```python
from build123d import *

# Parameters (mm, degrees)
F0_W     = 30
F0_H     = 30
F1_DEPTH = 15
F2_R     = 2
F4_R     = 1.75


with BuildPart() as f1:
    # F0 (on Top) → F1 (new body, symmetric)
    with BuildSketch(Plane.XY):
        Rectangle(F0_W, F0_H)
    extrude(amount=F1_DEPTH, both=True)

    # F2
    f2_edges = [f1.edges().sort_by_distance(p)[0] for p in [
        (15, 0, 15),
        (0, 15, 15),
        (-15, 0, 15),
        (0, -15, 15),
        (0, -15, -15),
        (15, -15, 0),
        (-15, -15, 0),
        (15, 0, -15),
        (15, 15, 0),
        (0, 15, -15),
        (-15, 15, 0),
        (-15, 0, -15),
    ]]
    fillet(f2_edges, radius=F2_R)

    # F5: sweep along a path in F3
    with BuildLine(Plane.XY) as f5_path:
        CenterArc((0, 19), 7, 0, 360)
    # F4 (on face) → F5 (sweep)
    with BuildSketch(Plane(origin=(0, 15, 0), x_dir=(-1, 0, 0), z_dir=(0, 1, 0))):
        with Locations((5.6, 0)):
            Circle(F4_R)
    sweep(path=f5_path.line)


solid = f1.part
```
Geometry: final body of the model. Coordinates: model frame, mm. Coordinates: 2 decimals unless noted, no trailing zeros. Write each loop counter-clockwise with the first axis right and the second up, starting at its lowest first coordinate (ties: lowest second). Pieces come first, ordered by that corner, then holes. Notation, with made-up numbers: M 39,60 L 62,60 A16 ccw 62,83 Z; hole C -38,-5 d1. An arc over 180 degrees is marked long. Answer as CSV lines item,"result". Start each with the question number.
Q1. Line query: line 1 (Y direction, x = -7.25, z = -9.25); line 2 (Y direction, x = -4, z = 0.5); line 3 (Y direction, x = -1.5, z = 13.5). Output: solid intervals per line, ascending. Write a range as from..to.
Q2. Pin query (flat end, axial travel): P1, Ø3, axis at x = 4, z = -10.5, coming from the +Y side. Return the tip coordinate at first contact, or that it passes through.
Q3. Cut plane A-A on z = 3.5. Return the cut outline in (x, y), then the cut area to 3 significant figures.
Findings below:
1,line 1,"y = -15..15"
1,line 2,"y = -15..15.08, 22.92..26.28"
1,line 3,"y = -14.94..14.94"
2,P1,"stops at y = 15"
3,outline,"M -15,-13 A2 ccw -13,-15 L 13,-15 A2 ccw 15,-13 L 15,13 A2 ccw 13,15 L -13,15 A2 ccw -15,13 Z"
3,area,"897 mm2"
